CAD build for the part. Positions are in the model's coordinates, mm. Face numbers are marked on the shaded views. A direction names the side the tool comes from. Coordinates: 2 decimals unless noted, no trailing zeros. Loops run counter-clockwise (first coordinate to the right, second up) from the corner with the lowest first, then second, coordinate; pieces in that order, holes last. Notation, with made-up numbers: (5.25, 61) - (38.25, 61) arc R20 cw to (38.25, 86) - close; hole circle Ø5 at (-1.75, 44). An arc over 180 degrees is marked (long way). Put each result on its own line as item: value.
```python
from build123d import *

# Parameters (mm, degrees)
F0_W     = 100
F0_H     = 150
F1_DEPTH = 3
F2_W     = 36
F2_H     = 36
F3_DEPTH = 200
F4_W     = 40
F4_H     = 120
F5_DEPTH = 25


with BuildPart() as f1:
    # F0 (on Front) → F1 (new body)
    with BuildSketch(Plane.XZ):
        Rectangle(F0_W, F0_H)
    extrude(amount=F1_DEPTH)

    # F2 (on face) → F3 (join)
    with BuildSketch(Plane.XZ.offset(3)):
        Polygon((20, 75), (0, 75), (-20, 75), (-20, 35), (20, 35), align=None)
        with Locations((0, 55)):
            Rectangle(F2_W, F2_H, mode=Mode.SUBTRACT)
    extrude(amount=F3_DEPTH)

    # F4 (on face) → F5 (join)
    with BuildSketch(Plane.XZ.offset(203)):
        with Locations((0, 15)):
            Rectangle(F4_W, F4_H)
    extrude(amount=F5_DEPTH)


solid = f1.part
```
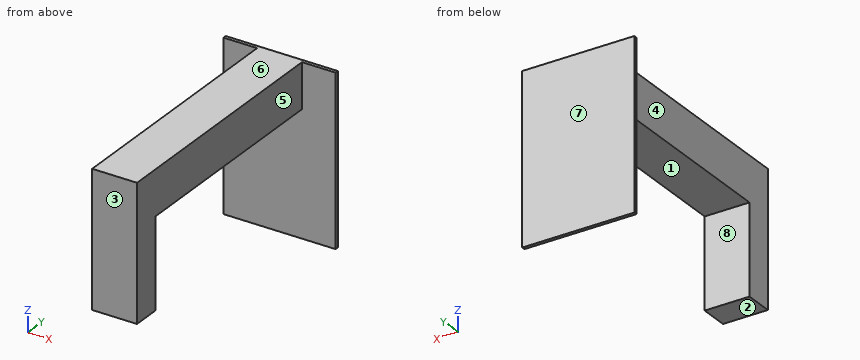
Q1. Wall check: L1, parallel to Y at x = -6, z = 19.5; L2, parallel to X at y = -150, z = 50.5; L3, parallel to Z at x = -8, y = -188.5. Give the ranges that are in metal, low to high. Write a range as from..to.
Determined:
L1: -228..-203, -3..0
L2: -20..-18, 18..20
L3: 35..37, 73..75
Q2. Mould opens along Y. For the marked faces 1, 2 and 3 say: +Y half, -Y half, draft (parallel to the pull), parting line (faces both ways), or undercut.
Determined:
face 1: undercut
face 2: draft
face 3: -Y half
Q3. Tool access for the marked faces 4, 5, 6, 7 and 8: list every direction of +Z, -Z, +X, -X, +Y, -Y with a clear straight run to the whole face (end or side of a thin tool).
Determined:
face 4: +Z, -Z, -X, -Y
face 5: +Z, -Z, +X, -Y
face 6: +Z, +X, -X, +Y, -Y
face 7: +Z, -Z, +X, -X, +Y
face 8: -Z, +X, -X
Q4. Slice it at D-D, the plane z = -54. Give the cut face in (x, y), then the cut area to 3 significant figures.
Determined:
outline: (-50, -3) - (50, -3) - (50, 0) - (-50, 0) - close
area: 300 mm2
Q5. Slice it at C-C, the plane x = -6. Give the cut face in (y, z).
Determined:
outline: (-228, -45) - (-203, -45) - (-203, 35) - (-3, 35) - (-3, -75) - (0, -75) - (0, 75) - (-228, 75) - close; hole (-203, 37) - (-3, 37) - (-3, 73) - (-203, 73) - close
Q6. Slice it at A-A, the plane y = -68. Give the cut face in (x, z).
Determined:
outline: (-20, 35) - (20, 35) - (20, 75) - (-20, 75) - close; hole (-18, 37) - (18, 37) - (18, 73) - (-18, 73) - close
Q7. Slice it at B-B, the plane z = -30.5. Give the cut face in (x, y).
Determined:
outline: (-50, -3) - (50, -3) - (50, 0) - (-50, 0) - close; (-20, -228) - (20, -228) - (20, -203) - (-20, -203) - close
Q8. Pin check, flat tips, straight feed: pin 1 Ø12 at (x, y) = (9, -126.5) entering from -Z; pin 2 Ø2 at (y, z) = (-180, 47.5) entering from +X; pin 3 Ø2 at (x, z) = (25.5, 48.5) entering from -Y; pin 4 Ø2 at (x, z) = (-11, -21) entering from +Y. Stop position of each tip, or through.
Determined:
pin 1: z = 35
pin 2: x = 20
pin 3: y = -3
pin 4: y = 0
